Input: dimensioned drawing with shaded views. Units: mm. Origin: part minimum x, y, z. A direction names the side the tool comes from. Give positions to 0.01 mm unless a question says otherwise; leave off trailing zeros. Loops run counter-clockwise (first coordinate to the right, second up) from the corner with the lowest first, then second, coordinate; pieces in that order, holes last.
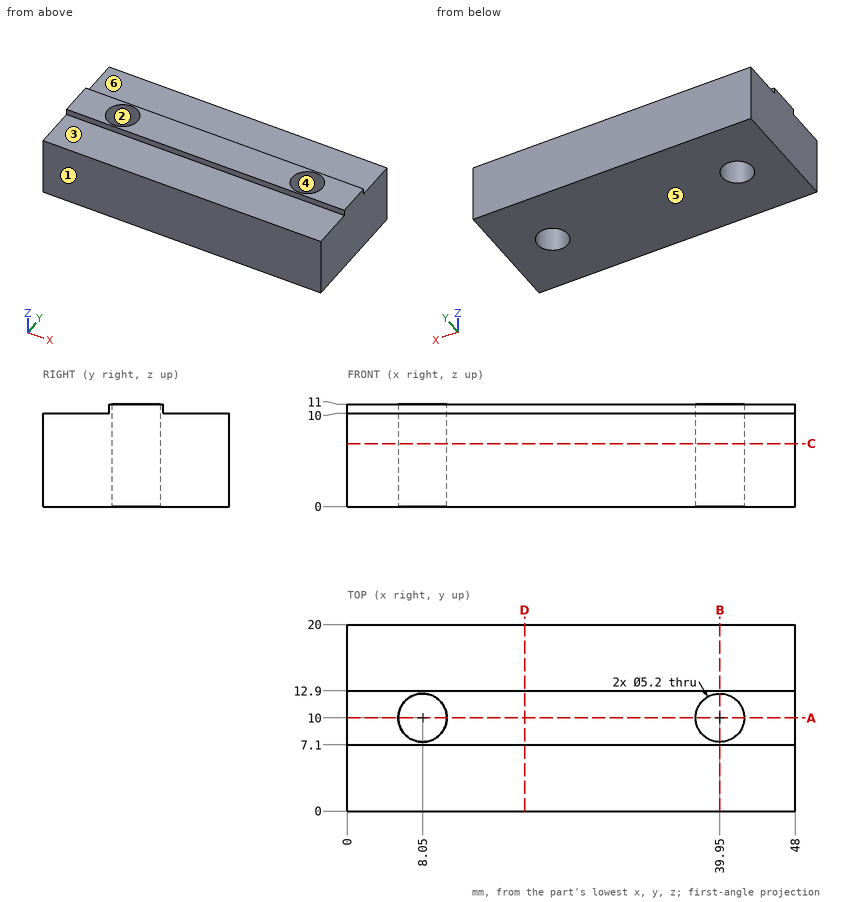
Item 1: Pin query (flat end, axial travel): pin 1 (2 mm diameter, centred on x = 17.5, y = 18, fed in from +Z); pin 2 (4 mm diameter, centred on x = 8.05, y = 10, fed in from -Z); pin 3 (1.5 mm diameter, centred on x = 37, y = 16, fed in from -Z); pin 4 (0.5 mm diameter, centred on x = 31, z = 10.5, fed in from +Y). Return the tip coordinate at first contact, or that it passes through.
Values follow:
pin 1: stops at z = 10
pin 2: passes through
pin 3: stops at z = 0
pin 4: stops at y = 12.9
Item 2: Section query A-A on y = 10. Return loops of the section in (x, z), plus the area to 3 significant figures.
Values follow:
outline: (0, 0) - (5.45, 0) - (5.45, 11) - (0, 11) - close; (10.65, 0) - (37.35, 0) - (37.35, 11) - (10.65, 11) - close; (42.55, 0) - (48, 0) - (48, 11) - (42.55, 11) - close
area: 414 mm2
Item 3: Ray query, probe 1 along Y at (x, z) = (39.95, 4.5); probe 2 along Z at (x, y) = (11, 7); probe 3 along Y at (x, z) = (38.5, 5.5). Return the intervals inside material, ascending.
Values follow:
probe 1: y = 0 to 7.4, 12.6 to 20
probe 2: z = 0 to 10
probe 3: y = 0 to 7.84, 12.16 to 20
Item 4: Draft query along Y for the marked faces 1, 2, 3 and 4. Return one class per face: +Y half, -Y half, draft (parallel to the pull), parting line (faces both ways), or undercut.
Values follow:
face 1: -Y half
face 2: undercut
face 3: draft
face 4: undercut
Item 5: Section query C-C on z = 6.75. Return loops of the section in (x, y).
Values follow:
outline: (0, 0) - (48, 0) - (48, 20) - (0, 20) - close; hole circle Ø5.2 at (8.05, 10); hole circle Ø5.2 at (39.95, 10)
Item 6: Set-up query: the marked faces 5 and 6. Return all of +Z, -Z, +X, -X, +Y, -Y with unobstructed straight access to the full face (end or side cutting, diameter ignored); none if empty.
Values follow:
face 5: -Z, +X, -X, +Y, -Y
face 6: +Z, +X, -X, +Y
Item 7: Section query B-B on x = 39.95. Return loops of the section in (y, z), plus the area to 3 significant figures.
Values follow:
outline: (0, 0) - (7.4, 0) - (7.4, 11) - (7.1, 11) - (7.1, 10) - (0, 10) - close; (12.6, 0) - (20, 0) - (20, 10) - (12.9, 10) - (12.9, 11) - (12.6, 11) - close
area: 149 mm2
Item 8: Section query D-D on x = 19. Return loops of the section in (y, z), plus the area to 3 significant figures.
Values follow:
outline: (0, 0) - (20, 0) - (20, 10) - (12.9, 10) - (12.9, 11) - (7.1, 11) - (7.1, 10) - (0, 10) - close
area: 206 mm2
